Answer from the drawing. Dimensions are ordinates in mm from the lowest x, y and z of the part. A direction names the side the tool comes from. Coordinates: 2 decimals unless noted, no trailing zeros. Write each loop counter-clockwise with the first axis right and the second up, starting at its lowest first coordinate (ties: lowest second). Pieces come first, ordered by that corner, then holes. Notation, with made-up numbers: (16, 20) -> (41, 20) arc R14 ccw to (41, 47) -> close; hole circle Ø4 at (61.5, 13). An arc over 180 degrees is marked (long way). Return JSON: item names as keys, results as strings.
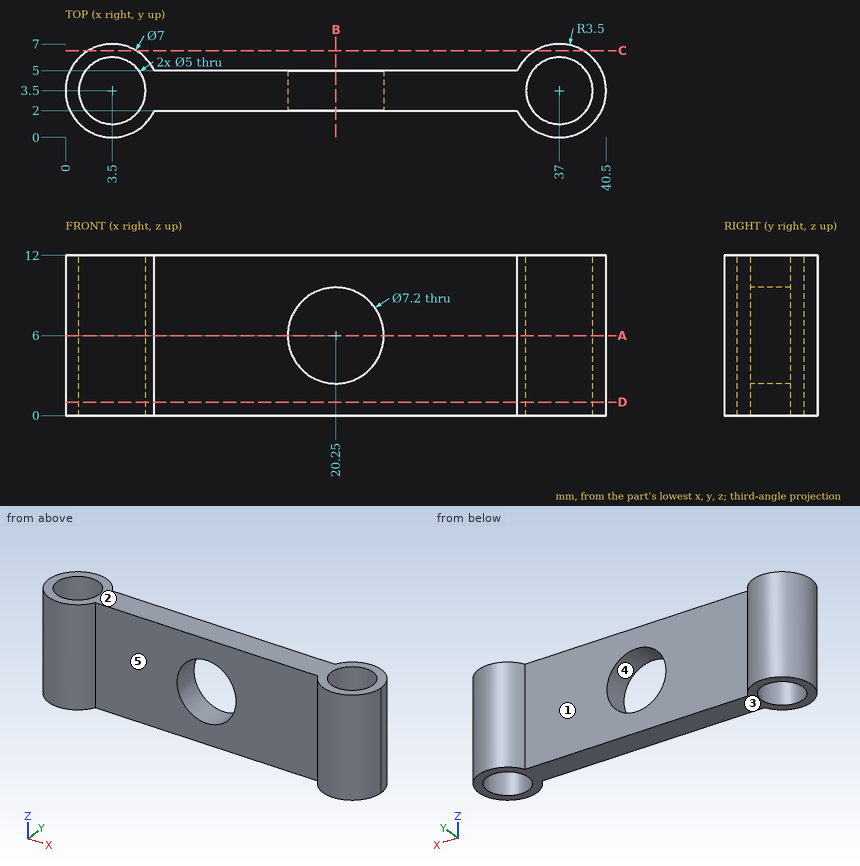
1. The part is cut by section D-D (z = 1). Determine the outline of the cut face in (x, y).
Taken from the geometry:
{"outline": "(6.66, 2) -> (33.84, 2) arc R3.5 ccw (long way) to (33.84, 5) -> (6.66, 5) arc R3.5 ccw (long way) to start; hole circle Ø5 at (3.5, 3.5); hole circle Ø5 at (37, 3.5)"}
2. The part is cut by section C-C (y = 6.5). Determine the outline of the cut face in (x, z).
Taken from the geometry:
{"outline": "(1.7, 0) -> (5.3, 0) -> (5.3, 12) -> (1.7, 12) -> close; (35.2, 0) -> (38.8, 0) -> (38.8, 12) -> (35.2, 12) -> close"}
3. The part is cut by section B-B (x = 20.25). Determine the outline of the cut face in (y, z), then the cut area to 3 significant figures.
Taken from the geometry:
{"outline": "(2, 0) -> (5, 0) -> (5, 2.4) -> (2, 2.4) -> close; (2, 9.6) -> (5, 9.6) -> (5, 12) -> (2, 12) -> close", "area": "14.4 mm2"}
4. The part is cut by section A-A (z = 6). Determine the outline of the cut face in (x, y), then the cut area to 3 significant figures.
Taken from the geometry:
{"outline": "(6.66, 2) -> (16.65, 2) -> (16.65, 5) -> (6.66, 5) arc R3.5 ccw (long way) to start; (23.85, 2) -> (33.84, 2) arc R3.5 ccw (long way) to (33.84, 5) -> (23.85, 5) -> close; hole circle Ø5 at (3.5, 3.5); hole circle Ø5 at (37, 3.5)", "area": "96.3 mm2"}
5. Consider L1, parallel to Z at x = 20.25, y = 3; L2, parallel to Y at x = 3.5, z = 6.5; L3, parallel to X at y = 2.75, z = 6.5. Determine where each line is inside the solid, lowest interval first.
Taken from the geometry:
{"L1": "z = 0 to 2.4, 9.6 to 12", "L2": "y = 0 to 1, 6 to 7", "L3": "x = 0.08 to 1.12, 5.88 to 16.68, 23.82 to 34.62, 39.38 to 40.42"}
6. A tool of negligible diameter and unlimited length cuts with its end or side. For the marked faces 1 and 2, from which of +Z, -Z, +X, -X, +Y, -Y can it reach the whole face along a straight path? Write none if from no direction.
Taken from the geometry:
{"face 1": "+Z, -Z, +Y", "face 2": "+Z, +X, -X, +Y, -Y"}
7. For a pull along X with two mould halves and no side action, classify the marked faces 3, 4 and 5 as +X half, -X half, draft (parallel to the pull), parting line (faces both ways), or undercut.
Taken from the geometry:
{"face 3": "draft", "face 4": "undercut", "face 5": "undercut"}
8. Flat-ended cylindrical pins translate along their axes: pin 1 Ø4 at (x, z) = (20.5, 9.5) entering from +Y; pin 2 Ø6 at (x, z) = (20, 8) entering from -Y; pin 3 Ø2 at (y, z) = (5.5, 8.5) entering from +X. Find the tip coordinate at first contact, or state that the pin passes through.
Taken from the geometry:
{"pin 1": "stops at y = 5", "pin 2": "stops at y = 2", "pin 3": "stops at x = 40.35"}
